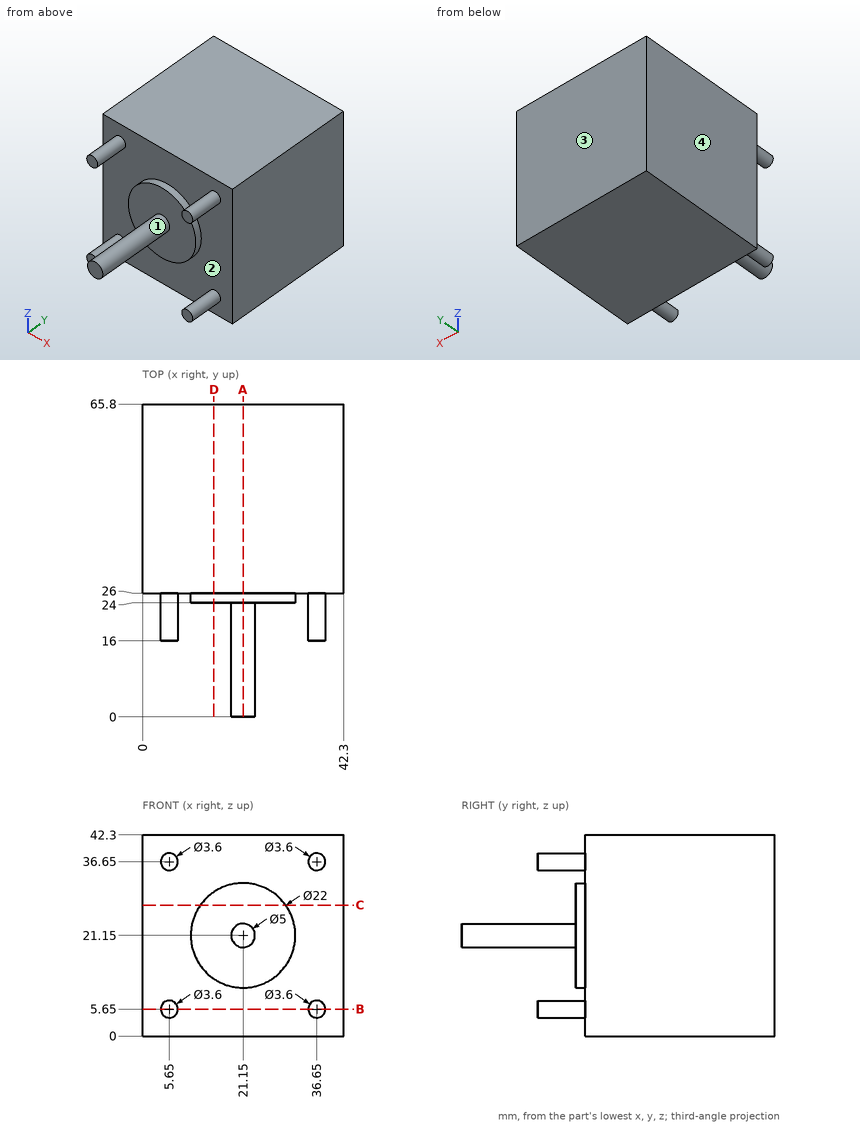
Source: three-view drawing plus pictorial views. Frame: mm from the lowest corner of the part. Give positions to 0.01 mm unless a question says otherwise; leave off trailing zeros. Order: outer loops, then holes, each group sorted by start corner. A loop starts at its lowest first (then second) coordinate and runs counter-clockwise, first axis right, second up. Notation, with made-up numbers: (6.25, 19) -> (52.25, 19) arc R18 ccw to (52.25, 45) -> close; hole circle Ø11 at (-14, 25). An arc over 180 degrees is marked (long way). Write each question's results on one line, items separated by ' | '. Start each with the question number.
Item 1: Cut plane C-C on z = 27.5. Return the cut outline in (x, y), then the cut area to 3 significant figures.
Item 2: Contact query for flat-ended pins moving along their axis: P1, Ø4, axis at y = 19, z = 15.5, coming from the -X side; P2, Ø4, axis at x = 36, z = 37.5, coming from the -Y side; P3, Ø5, axis at y = 37, z = 23, coming from the -X side; P4, Ø1, axis at x = 15, z = 24, coming from the -Y side. Output: stop coordinate, or through.
Item 3: Cut plane D-D on x = 15. Return the cut outline in (y, z), then the cut area to 3 significant figures.
Item 4: Cut plane A-A on x = 21.15. Return the cut outline in (y, z).
Item 5: Line query: line 1 (Y direction, x = 14.5, z = 5); line 2 (Y direction, x = 17, z = 21.5); line 3 (X direction, y = 10, z = 20.5). Output: solid intervals per line, ascending.
Item 6: Cut plane B-B on z = 5.65. Return the cut outline in (x, y), then the cut area to 3 significant figures.
Item 7: Mould query, pull axis X, two halves, no side actions, for the marked faces 1, 2, 3 and 4. Classes: pulls with the +X half, pulls with the -X half, needs draft (parallel to the pull), parting line crosses it, or undercut.
Established:
1) outline: (0, 26) -> (12.17, 26) -> (12.17, 24) -> (30.13, 24) -> (30.13, 26) -> (42.3, 26) -> (42.3, 65.8) -> (0, 65.8) -> close | area: 1,720 mm^2
2) P1: through | P2: y = 16 | P3: x = 0 | P4: y = 24
3) outline: (24, 12.03) -> (26, 12.03) -> (26, 0) -> (65.8, 0) -> (65.8, 42.3) -> (26, 42.3) -> (26, 30.27) -> (24, 30.27) -> close | area: 1,720 mm^2
4) outline: (0, 18.65) -> (24, 18.65) -> (24, 10.15) -> (26, 10.15) -> (26, 0) -> (65.8, 0) -> (65.8, 42.3) -> (26, 42.3) -> (26, 32.15) -> (24, 32.15) -> (24, 23.65) -> (0, 23.65) -> close
5) line 1: 26 to 65.8 | line 2: 24 to 65.8 | line 3: 18.74 to 23.56
6) outline: (0, 26) -> (3.85, 26) -> (3.85, 16) -> (7.45, 16) -> (7.45, 26) -> (34.85, 26) -> (34.85, 16) -> (38.45, 16) -> (38.45, 26) -> (42.3, 26) -> (42.3, 65.8) -> (0, 65.8) -> close | area: 1,760 mm^2
7) face 1: parting line crosses it | face 2: undercut | face 3: needs draft | face 4: pulls with the -X half
